Input: part model. Units: mm. Frame: model coordinates. A direction names the side the tool comes from. Give positions to 0.01 mm unless a question says otherwise; leave off trailing zeros. Loops run counter-clockwise (first coordinate to the right, second up) from the corner with the lowest first, then second, coordinate; pieces in that order, holes last. Notation, with made-up numbers: (57.25, 80) -> (64.25, 80) arc R12 cw to (64.25, 100) -> close; hole circle Ø2 at (-21.5, 58). An arc over 180 degrees is marked (long way). Answer as a JSON object with one key per item and string values.
```python
from build123d import *

# Parameters (mm, degrees)
SKETCH1_R           = 5
BOSS_EXTRUDE1_DEPTH = 4


with BuildPart() as part:
    # Sketch1 → Boss-Extrude1 (new body)
    with BuildSketch(Plane.XY):
        Polygon((-46, 5), (-46, 15), (-42, 15), (-42, 25), (42, 25), (42, 15), (46, 15), (46, 5), (42, 5), (42, -5), (46, -5), (46, -15), (42, -15), (42, -25), (-42, -25), (-42, -15), (-46, -15), (-46, -5), (-42, -5), (-42, 5), align=None)
        Circle(SKETCH1_R, mode=Mode.SUBTRACT)
    extrude(amount=BOSS_EXTRUDE1_DEPTH)


solid = part.part
```
Q1. Section D-D, the plane y = 21. Return the cut outline in (x, z), then the cut area to 3 significant figures.
Evaluation:
{"outline": "(-42, 0) -> (42, 0) -> (42, 4) -> (-42, 4) -> close", "area": "336 mm2"}
Q2. Section B-B, the plane y = 0. Return the cut outline in (x, z).
Evaluation:
{"outline": "(-42, 0) -> (-5, 0) -> (-5, 4) -> (-42, 4) -> close; (5, 0) -> (42, 0) -> (42, 4) -> (5, 4) -> close"}
Q3. Access query for faces 1 (the flat face through (-42, 0, 2)), 2 (the flat face through (42, 20, 2)), 3 (the flat face through (44, 5, 2)), 4 (the flat face through (-44, 15, 2)). Directions: +Z, -Z, +X, -X, +Y, -Y. A direction counts if a zero-diameter tool reaches every point of the face in a straight line with its end or side. Return the directions, or none.
Evaluation:
{"face 1": "+Z, -Z, -X", "face 2": "+Z, -Z, +X, +Y", "face 3": "+Z, -Z, +X", "face 4": "+Z, -Z, -X, +Y"}
Q4. Ray query, line 1 along Y through (x, z) = (0, 1.3); line 2 along X through (y, z) = (-18, 0.5); line 3 along Y through (x, z) = (42.5, 1.75). Return the intervals inside material, ascending.
Evaluation:
{"line 1": "y = -25 to -5, 5 to 25", "line 2": "x = -42 to 42", "line 3": "y = -15 to -5, 5 to 15"}
Q5. Draft query along Y for faces 5 (the cylindrical face through (-1.08, -4.88, 1.97)), 6 (the flat face through (44, -15, 2)), 7 (the flat face through (44, 15, 2)), 8 (the flat face through (-42, 20, 2)). Return one class per face: +Y half, -Y half, draft (parallel to the pull), parting line (faces both ways), or undercut.
Evaluation:
{"face 5": "undercut", "face 6": "-Y half", "face 7": "+Y half", "face 8": "draft"}
Q6. Pin query (flat end, axial travel): pin 1 (8 mm diameter, centred on x = 0, y = 4, fed in from +Z); pin 2 (1.2 mm diameter, centred on x = -45, z = 2, fed in from +Y); pin 3 (1.2 mm diameter, centred on y = -21.5, z = 1, fed in from +X); pin 4 (1.2 mm diameter, centred on y = 18.5, z = 1.5, fed in from -X). Return the tip coordinate at first contact, or that it passes through.
Evaluation:
{"pin 1": "stops at z = 4", "pin 2": "stops at y = 15", "pin 3": "stops at x = 42", "pin 4": "stops at x = -42"}
Q7. Section C-C, the plane x = 0. Return the cut outline in (y, z), then the cut area to 3 significant figures.
Evaluation:
{"outline": "(-25, 0) -> (-5, 0) -> (-5, 4) -> (-25, 4) -> close; (5, 0) -> (25, 0) -> (25, 4) -> (5, 4) -> close", "area": "160 mm2"}
Q8. Section A-A, the plane z = 0.9. Return the cut outline in (x, y), then the cut area to 3 significant figures.
Evaluation:
{"outline": "(-46, -15) -> (-42, -15) -> (-42, -25) -> (42, -25) -> (42, -15) -> (46, -15) -> (46, -5) -> (42, -5) -> (42, 5) -> (46, 5) -> (46, 15) -> (42, 15) -> (42, 25) -> (-42, 25) -> (-42, 15) -> (-46, 15) -> (-46, 5) -> (-42, 5) -> (-42, -5) -> (-46, -5) -> close; hole circle Ø10 at (0, 0)", "area": "4,280 mm2"}
